Design review of the part built by this model. Coordinates are the model's own, in mm. A direction names the side the tool comes from. Give positions to 0.01 mm unless a question says otherwise; leave off trailing zeros.
```python
from build123d import *

# Parameters (mm, degrees)
SKETCH_1_W          = 85
SKETCH_1_H          = 85
EXTRUDE_1_DEPTH     = 2
CUT_EXTRUDE_1_DEPTH = 3
SKETCH_4_R          = 1.5
CUT_EXTRUDE_2_DEPTH = 3
SKETCH_5_R          = 1.5
CUT_EXTRUDE_3_DEPTH = 2
SKETCH_6_W          = 37
SKETCH_6_H          = 3
SKETCH_6_W_2        = 3
SKETCH_6_H_2        = 37
SKETCH_6_W_3        = 11.313708498
SKETCH_6_H_3        = 11.313708498
CUT_EXTRUDE_4_DEPTH = 2


with BuildPart() as part:
    # 草图1 → 凸台-拉伸1 (new body)
    with BuildSketch(Plane.XY):
        with Locations((42.5, 42.5)):
            Rectangle(SKETCH_1_W, SKETCH_1_H)
    extrude(amount=EXTRUDE_1_DEPTH)

    # 草图2 → 切除-拉伸1 (cut)
    with BuildSketch(Plane.XY):
        Polygon((0, 85), (14, 85), (0, 71), align=None)
        Polygon((0, 0), (14, 0), (0, 14), align=None)
        Polygon((85, 85), (71, 85), (85, 71), align=None)
        Polygon((85, 0), (85, 14), (71, 0), align=None)
    extrude(amount=CUT_EXTRUDE_1_DEPTH, mode=Mode.SUBTRACT)

    # 草图4 → 切除-拉伸2 (cut)
    with BuildSketch(Plane.XY):
        with Locations(Location((13.292893219, 80.050252532, 0), (0, 0, 180))):
            Circle(SKETCH_4_R)
        with Locations(Location((4.949747468, 71.707106781, 0), (0, 0, 180))):
            Circle(SKETCH_4_R)
        with Locations(Location((10.253048327, 69.232233047, 0), (0, 0, 180))):
            Circle(SKETCH_4_R)
        with Locations(Location((15.767766953, 74.746951673, 0), (0, 0, 180))):
            Circle(SKETCH_4_R)
        with Locations(Location((4.949747468, 13.292893219, 0), (0, 0, 180))):
            Circle(SKETCH_4_R)
        with Locations(Location((13.292893219, 4.949747468, 0), (0, 0, 180))):
            Circle(SKETCH_4_R)
        with Locations(Location((10.253048327, 15.767766953, 0), (0, 0, 180))):
            Circle(SKETCH_4_R)
        with Locations(Location((15.767766953, 10.253048327, 0), (0, 0, 180))):
            Circle(SKETCH_4_R)
        with Locations(Location((71.707106781, 4.949747468, 0), (0, 0, 180))):
            Circle(SKETCH_4_R)
        with Locations(Location((69.232233047, 10.253048327, 0), (0, 0, 180))):
            Circle(SKETCH_4_R)
        with Locations(Location((75.100505063, 15.414213562, 0), (0, 0, 180))):
            Circle(SKETCH_4_R)
        with Locations(Location((80.050252532, 13.292893219, 0), (0, 0, 180))):
            Circle(SKETCH_4_R)
        with Locations(Location((71.707106781, 80.050252532, 0), (0, 0, 180))):
            Circle(SKETCH_4_R)
        with Locations(Location((69.232233047, 74.746951673, 0), (0, 0, 180))):
            Circle(SKETCH_4_R)
        with Locations(Location((74.746951673, 69.232233047, 0), (0, 0, 180))):
            Circle(SKETCH_4_R)
        with Locations(Location((80.050252532, 71.707106781, 0), (0, 0, 180))):
            Circle(SKETCH_4_R)
    extrude(amount=CUT_EXTRUDE_2_DEPTH, mode=Mode.SUBTRACT)

    # 草图5 → 切除-拉伸3 (cut)
    with BuildSketch(Plane.XY):
        with Locations((8, 61)):
            Circle(SKETCH_5_R)
        with Locations((8, 24)):
            Circle(SKETCH_5_R)
        with Locations((24, 8)):
            Circle(SKETCH_5_R)
        with Locations((61, 8)):
            Circle(SKETCH_5_R)
        with Locations((77, 24)):
            Circle(SKETCH_5_R)
        with Locations((77, 61)):
            Circle(SKETCH_5_R)
        with Locations((61, 77)):
            Circle(SKETCH_5_R)
        with Locations((24, 77)):
            Circle(SKETCH_5_R)
    extrude(amount=CUT_EXTRUDE_3_DEPTH, mode=Mode.SUBTRACT)

    # 草图6 → 切除-拉伸4 (cut)
    with BuildSketch(Plane.XY):
        with Locations((42.5, 17.267766953)):
            Rectangle(SKETCH_6_W, SKETCH_6_H)
        with Locations((42.5, 67.732233047)):
            Rectangle(SKETCH_6_W, SKETCH_6_H)
        with Locations((17.267766953, 42.5)):
            Rectangle(SKETCH_6_W_2, SKETCH_6_H_2)
        with Locations((67.732233047, 42.5)):
            Rectangle(SKETCH_6_W_2, SKETCH_6_H_2)
        with BuildLine():
            Line((26.899494937, 60.221825407), (33.970562748, 53.150757595))
            ThreePointArc((33.970562748, 53.150757595), (33.970562748, 51.029437252), (31.849242405, 51.029437252))
            Line((31.849242405, 51.029437252), (24.778174593, 58.100505063))
            ThreePointArc((24.778174593, 58.100505063), (24.778174593, 60.221825407), (26.899494937, 60.221825407))
        make_face()
        with BuildLine():
            Line((24.778174593, 26.899494937), (31.849242405, 33.970562748))
            ThreePointArc((31.849242405, 33.970562748), (33.970562748, 33.970562748), (33.970562748, 31.849242405))
            Line((33.970562748, 31.849242405), (26.899494937, 24.778174593))
            ThreePointArc((26.899494937, 24.778174593), (24.778174593, 24.778174593), (24.778174593, 26.899494937))
        make_face()
        with BuildLine():
            Line((60.221825407, 58.100505063), (53.150757595, 51.029437252))
            ThreePointArc((53.150757595, 51.029437252), (51.029437252, 51.029437252), (51.029437252, 53.150757595))
            Line((51.029437252, 53.150757595), (58.100505063, 60.221825407))
            ThreePointArc((58.100505063, 60.221825407), (60.221825407, 60.221825407), (60.221825407, 58.100505063))
        make_face()
        with BuildLine():
            Line((58.100505063, 24.778174593), (51.029437252, 31.849242405))
            ThreePointArc((51.029437252, 31.849242405), (51.029437252, 33.970562748), (53.150757595, 33.970562748))
            Line((53.150757595, 33.970562748), (60.221825407, 26.899494937))
            ThreePointArc((60.221825407, 26.899494937), (60.221825407, 24.778174593), (58.100505063, 24.778174593))
        make_face()
        with Locations((42.5, 42.5)):
            Rectangle(SKETCH_6_W_3, SKETCH_6_H_3)
    extrude(amount=CUT_EXTRUDE_4_DEPTH, mode=Mode.SUBTRACT)


solid = part.part
```
1. For line 1 along Y through (x, z) = (35, 0.3); line 2 along X through (y, z) = (48, 1.8), list the stretches that pass through material, from the lowest coordinate up.
Recorded:
line 1: y = 0 to 15.77, 18.77 to 66.23, 69.23 to 85
line 2: x = 0 to 15.77, 18.77 to 36.84, 48.16 to 66.23, 69.23 to 85
2. Machinability: for faces 1 (the face through (56.736, 54.614, 0.986)), 2 (the face through (7, 7, 1)), which of the approach directions +Z, -Z, +X, -X, +Y, -Y give a long, thin tool a straight path to every point of the face, cutting with its end or side? Answer none if there is none.
Recorded:
face 1: +Z, -Z
face 2: +Z, -Z, -X, -Y
3. For pin 1 (5 mm diameter, centred on x = 13.29, y = 80.05, fed in from -Z); pin 2 (1 mm diameter, centred on y = 13, z = 1, fed in from -X); pin 3 (1.8 mm diameter, centred on x = 80.05, y = 13.29, fed in from -Z), all flat-tipped, find the tip position at first contact; note any pin that passes through.
Recorded:
pin 1: stops at z = 0
pin 2: stops at x = 0.5
pin 3: passes through
4. Draft analysis for pull direction Y (two halves, no side actions). For faces 3 (the face through (42, 0, 1)), 4 (the face through (42, 34, 2)), 5 (the face through (56.64, 30.48, 0.99)), state which applies: pulls with the +Y half, pulls with the -Y half, needs draft (parallel to the pull), parting line crosses it, or undercut.
Recorded:
face 3: pulls with the -Y half
face 4: needs draft
face 5: undercut
5. Take a section at A-A (z = 1.4). State how many separate pieces and enclosed holes the cut face has, then the cut area to 3 significant figures.
Recorded:
separate pieces: 1
enclosed holes: 33
area: 5,940 mm2
